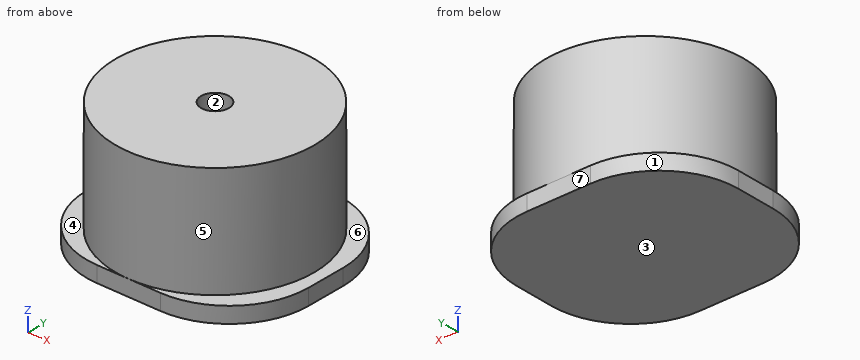
```python
from build123d import *

# Parameters (mm, degrees)
SKETCH_1_R          = 12.5
EXTRUDE_1_DEPTH     = 14
SKETCH_2_R          = 1.75
CUT_EXTRUDE_1_DEPTH = 6
SKETCH_3_W          = 28
SKETCH_3_H          = 25
EXTRUDE_2_DEPTH     = 2
FILLET_1_R          = 10


with BuildPart() as part:
    # ｽｹｯﾁ1 → ﾎﾞｽ - 押し出し1 (new body)
    with BuildSketch(Plane.XY):
        Circle(SKETCH_1_R)
    extrude(amount=EXTRUDE_1_DEPTH)

    # ｽｹｯﾁ2 → ｶｯﾄ - 押し出し1 (cut)
    with BuildSketch(Plane.XY.offset(14)):
        Circle(SKETCH_2_R)
    extrude(amount=-CUT_EXTRUDE_1_DEPTH, mode=Mode.SUBTRACT)

    # ｽｹｯﾁ3 → ﾎﾞｽ - 押し出し2 (add)
    with BuildSketch(Plane(origin=(0, 0, 0), x_dir=(-1, 0, 0), z_dir=(0, 0, -1))):
        Rectangle(SKETCH_3_W, SKETCH_3_H)
    extrude(amount=EXTRUDE_2_DEPTH)

    # ﾌｨﾚｯﾄ1
    fillet_1_edges = [part.edges().sort_by_distance(p)[0] for p in [
        (14, 12.5, -1),
        (14, -12.5, -1),
        (-14, -12.5, -1),
        (-14, 12.5, -1),
    ]]
    fillet(fillet_1_edges, radius=FILLET_1_R)


solid = part.part
```
Verification items for the finished model (mm, model axes). Face numbers are marked on the shaded views. A direction names the side the tool comes from. Round coordinates to 2 decimals unless told otherwise and drop trailing zeros. Write each loop counter-clockwise with the first axis right and the second up, starting at its lowest first coordinate (ties: lowest second). Pieces come first, ordered by that corner, then holes. Notation, with made-up numbers: (0.5, 37.25) -> (6.5, 37.25) arc R25 cw to (6.5, 76.25) -> close; hole circle Ø11 at (61, 79.5). An arc over 180 degrees is marked (long way). Write each question's results on one line, items separated by ' | '.
Q1. Thickness scan on probe 1 along Y at (x, z) = (0, 10.2); probe 2 along Y at (x, z) = (-0.25, 5); probe 3 along Y at (x, z) = (-0.75, 9.25). Record the ranges inside material, lowest first.
Derived:
probe 1: y = -12.5 to -1.75, 1.75 to 12.5 | probe 2: y = -12.5 to 12.5 | probe 3: y = -12.48 to -1.58, 1.58 to 12.48
Q2. Sectioned sample at D-D, the plane y = -4. Record the boundary of the cut face in (x, z).
Derived:
outline: (-13.89, -2) -> (13.89, -2) -> (13.89, 0) -> (11.84, 0) -> (11.84, 14) -> (-11.84, 14) -> (-11.84, 0) -> (-13.89, 0) -> close
Q3. Sectioned sample at C-C, the plane x = 3.25. Record the boundary of the cut face in (y, z), and give its area (3 significant figures).
Derived:
outline: (-12.5, -2) -> (12.5, -2) -> (12.5, 0) -> (12.07, 0) -> (12.07, 14) -> (-12.07, 14) -> (-12.07, 0) -> (-12.5, 0) -> close | area: 388 mm²
Q4. Access from +Z, -Z, +X, -X, +Y, -Y to the whole of each face (thin tool, end or side, straight path). Record for the marked faces 4, 5, 6 and 7.
Derived:
face 4: +Z, -X | face 5: +Z | face 6: +Z, +X | face 7: +Z, -Z, +X, -X, +Y
Q5. Draft check along Y on the marked faces 1, 2 and 3. Enter one of: released by +Y, released by -Y, zero draft, split by the parting line, or undercut.
Derived:
face 1: released by +Y | face 2: undercut | face 3: zero draft
Q6. Sectioned sample at B-B, the plane z = 12.5. Record the boundary of the cut face in (x, y), and give its area (3 significant figures).
Derived:
outline: circle Ø25 at (0, 0); hole circle Ø3.5 at (0, 0) | area: 481 mm²
Q7. Go/stop test with flat-tipped pins: pin 1 Ø5 at (x, z) = (4.5, 4.5) entering from -Y; pin 2 Ø3 at (y, z) = (2.5, 8) entering from +X. Record where each tip stops, or that it passes through.
Derived:
pin 1: stops at y = -12.34 | pin 2: stops at x = 12.46
Q8. Sectioned sample at A-A, the plane y = 0. Record the boundary of the cut face in (x, z).
Derived:
outline: (-14, -2) -> (14, -2) -> (14, 0) -> (12.5, 0) -> (12.5, 14) -> (1.75, 14) -> (1.75, 8) -> (-1.75, 8) -> (-1.75, 14) -> (-12.5, 14) -> (-12.5, 0) -> (-14, 0) -> close
